Geometry check sheet. Reference: the model listing, model coordinates, mm. Round coordinates to 2 decimals unless told otherwise and drop trailing zeros. Write each loop counter-clockwise with the first axis right and the second up, starting at its lowest first coordinate (ties: lowest second). Pieces come first, ordered by that corner, then holes. Notation, with made-up numbers: (67, 75.25) -> (103, 75.25) arc R22 cw to (103, 96.25) -> close; hole circle Ø1 at (73.25, 12.25). An arc over 180 degrees is marked (long way). Return JSON: item names as keys, results as strings. Group by question number.
from build123d import *

# Parameters (mm, degrees)
SKETCH_1_W          = 80.5
SKETCH_1_H          = 162
SKETCH_1_R          = 1.525
EXTRUDE_1_DEPTH     = 1
SKETCH_2_R          = 97.5
CUT_EXTRUDE_1_DEPTH = 1
FILLET_1_R          = 2
EXTRUDE_2_DEPTH     = 1
FILLET_2_R          = 2
CUT_EXTRUDE_2_DEPTH = 10
FILLET_3_R          = 2


with BuildPart() as part:
    # 草图1 → 凸台-拉伸1 (new body)
    with BuildSketch(Plane.XY):
        with Locations((-4.75, 0)):
            Rectangle(SKETCH_1_W, SKETCH_1_H)
        with Locations((-10, 77)):
            Circle(SKETCH_1_R, mode=Mode.SUBTRACT)
        with Locations((10, 77)):
            Circle(SKETCH_1_R, mode=Mode.SUBTRACT)
        with Locations((-10, -77)):
            Circle(SKETCH_1_R, mode=Mode.SUBTRACT)
        with Locations((10, -77)):
            Circle(SKETCH_1_R, mode=Mode.SUBTRACT)
    extrude(amount=EXTRUDE_1_DEPTH)

    # 草图2 → 切除-拉伸1 (cut)
    with BuildSketch(Plane(origin=(0, 0, 0), x_dir=(-1, 0, 0), z_dir=(0, 0, -1))):
        with Locations((-111, 0)):
            Circle(SKETCH_2_R)
    extrude(amount=-CUT_EXTRUDE_1_DEPTH, mode=Mode.SUBTRACT)

    # 圆角1
    fillet_1_edges = [part.edges().sort_by_distance(p)[0] for p in [
        (35.5, -61.692787261, 0.5),
        (35.5, 61.692787261, 0.5),
        (35.5, -81, 0.5),
        (-45, -81, 0.5),
        (-45, 81, 0.5),
        (35.5, 81, 0.5),
    ]]
    fillet(fillet_1_edges, radius=FILLET_1_R)

    # 草图3 → 凸台-拉伸2 (add)
    with BuildSketch(Plane.XY.offset(1)):
        Polygon((-91, 81), (-91, 55.5), (-45, 55.5), (-45, 39.5), (-91, 39.5), (-91, -39.5), (-45, -39.5), (-45, -55.5), (-91, -55.5), (-91, -81), (-43, -81), (-43, 81), align=None)
    extrude(amount=-EXTRUDE_2_DEPTH)

    # 圆角2
    fillet_2_edges = [part.edges().sort_by_distance(p)[0] for p in [
        (-91, -81, 0.5),
        (-45, -55.5, 0.5),
        (-91, -55.5, 0.5),
        (-91, 55.5, 0.5),
        (-45, 55.5, 0.5),
        (-91, 81, 0.5),
        (-45, -39.5, 0.5),
        (-45, 39.5, 0.5),
        (-91, 39.5, 0.5),
        (-91, -39.5, 0.5),
    ]]
    fillet(fillet_2_edges, radius=FILLET_2_R)

    # 草图4 → 切除-拉伸2 (cut)
    with BuildSketch(Plane.XY.offset(1)):
        with BuildLine():
            Line((-47, 55.5), (-43, 55.5))
            Line((-43, 55.5), (-43, 39.5))
            Line((-43, 39.5), (-47, 39.5))
            ThreePointArc((-47, 39.5), (-45.585786438, 40.085786438), (-45, 41.5))
            Line((-45, 41.5), (-45, 53.5))
            ThreePointArc((-45, 53.5), (-45.585786438, 54.914213562), (-47, 55.5))
        make_face()
        with BuildLine():
            Line((-47, -39.5), (-43, -39.5))
            Line((-43, -39.5), (-43, -55.5))
            Line((-43, -55.5), (-47, -55.5))
            ThreePointArc((-47, -55.5), (-45.585786438, -54.914213562), (-45, -53.5))
            Line((-45, -53.5), (-45, -41.5))
            ThreePointArc((-45, -41.5), (-45.585786438, -40.085786438), (-47, -39.5))
        make_face()
    extrude(amount=-CUT_EXTRUDE_2_DEPTH, mode=Mode.SUBTRACT)

    # 圆角3
    fillet_3_edges = [part.edges().sort_by_distance(p)[0] for p in [
        (-43, 55.5, 0.5),
        (-43, 39.5, 0.5),
        (-43, -39.5, 0.5),
        (-43, -55.5, 0.5),
    ]]
    fillet(fillet_3_edges, radius=FILLET_3_R)


solid = part.part
1) Sectioned sample at C-C on y = 22.5. Enter the section's corners in (x, z).
2) Mould release check, pull along Y, two halves, no side actions. Record for faces 1 (the face through (13.504, -0.925, 0.493)), 2 (the face through (-29, 1, 1)): +Y half, -Y half, draft (parallel to the pull), parting line (faces both ways), or undercut.
3) Go/stop test with a flat-tipped pin: P1, Ø3.5, axis at x = 10, y = 77, coming from the -Z side. Record where the tip stops, or that it passes through.
4) Sectioned sample at A-A on x = -50. Enter the section's corners in (y, z), and give its area (3 significant figures).
5) Material ranges on probe 1 along X at (y, z) = (77, 0.8) (3 decimals); probe 2 along Y at (x, z) = (-59.5, 0.75); probe 3 along Y at (x, z) = (10, 0.7) (3 decimals), recorded low to high. Write a range as [from, to].
6) Sectioned sample at B-B on z = 0.8. State how many separate pieces and enclosed holes the cut face has, and give its area (3 significant figures).
Evaluation:
{
 "1": {"outline": "(-91, 0) -> (16.13, 0) -> (16.13, 1) -> (-91, 1) -> close"},
 "2": {"face 1": "undercut", "face 2": "draft"},
 "3": {"P1": "stops at z = 0"},
 "4": {"outline": "(-81, 0) -> (-55.5, 0) -> (-55.5, 1) -> (-81, 1) -> close; (-39.5, 0) -> (39.5, 0) -> (39.5, 1) -> (-39.5, 1) -> close; (55.5, 0) -> (81, 0) -> (81, 1) -> (55.5, 1) -> close", "area": "130 mm2"},
 "5": {"probe 1": "x = [-91, -11.525], [-8.475, 8.475], [11.525, 35.5]", "probe 2": "y = [-81, -55.5], [-39.5, 39.5], [55.5, 81]", "probe 3": "y = [-81, -78.525], [-75.475, 75.475], [78.525, 81]"},
 "6": {"separate pieces": "1", "enclosed holes": "4", "area": "17,100 mm2"}
}
